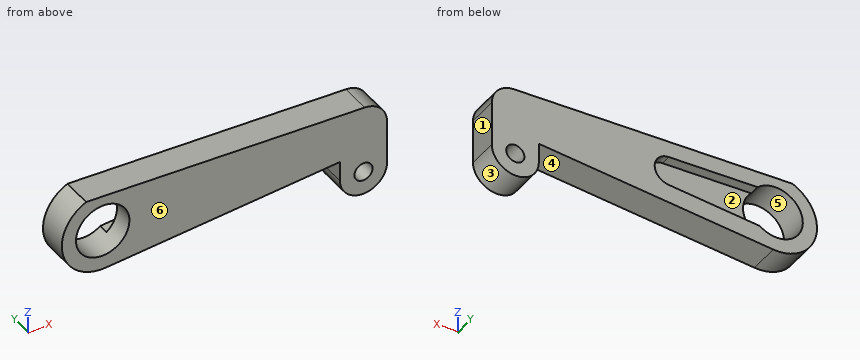
from build123d import *

# Parameters (mm, degrees)
BOSS_EXTRUDE1_START    = -1.35
BOSS_EXTRUDE1_DEPTH    = 1.35
SKETCH4_R              = 1.2192
BOSS_EXTRUDE2_DEPTH    = 4
BODY_DELETE1_OUTLINE_R = 2.45
BODY_DELETE1_DEPTH     = 4


# Read off the part's stored shape, not the designer's step: Body-Delete1
with BuildPart() as part:
    # Sketch2 → Revolve1 (revolve)
    with BuildSketch(Plane.XY, mode=Mode.PRIVATE) as revolve1_sk:
        Polygon((2.45, 0), (2.45, 2.25), (1.2, 2.25), (1.2, 3), (2.45, 3), (2.45, 4), (3.585, 4), (3.585, 0), align=None)
    revolve(revolve1_sk.sketch.rotate(Axis((0, 0, 0), (0, 1, 0)), 90), axis=Axis((0, 0, 0), (0, 1, 0)))

    # Sketch3 → Boss-Extrude1 (add)
    with BuildSketch(Plane(origin=(0, 4, 0), x_dir=(1, 0, 0), z_dir=(0, 1, 0)).offset(BOSS_EXTRUDE1_START)):
        with BuildLine():
            Line((2.174793094, 2.85), (14.4288372, 1.998853492))
            ThreePointArc((14.4288372, 1.998853492), (16.293577458, -0.019194273), (14.390517199, -2.001146508))
            Line((14.390517199, -2.001146508), (2.468243302, -2.6))
            ThreePointArc((2.468243302, -2.6), (3.579814485, 0.1927518), (2.174793094, 2.85))
        make_face()
    extrude(amount=BOSS_EXTRUDE1_DEPTH)


with BuildPart() as body_2:
    # Sketch4 → Boss-Extrude2 (new body)
    with BuildSketch(Plane(origin=(0, 0, 0), x_dir=(1, 0, 0), z_dir=(0, 1, 0))):
        with BuildLine():
            Line((0.380676568, 5.480639828), (31.845967375, 3.295110532))
            Line((31.845967375, 3.295110532), (31.845967375, 6))
            ThreePointArc((31.845967375, 6), (35, 9.154032625), (38.154032625, 6))
            Line((38.154032625, 6), (38.154032625, 0))
            ThreePointArc((38.154032625, 0), (37.285495002, -2.173576407), (35.158226963, -3.150061274))
            Line((35.158226963, -3.150061274), (-2.215454853, -5.027334022))
            ThreePointArc((-2.215454853, -5.027334022), (-5.333477425, 1.317704871), (0.380676568, 5.480639828))
        make_face()
        with Locations(Location((35, 6, 0), (0, 0, 270))):
            Circle(SKETCH4_R, mode=Mode.SUBTRACT)
    extrude(amount=BOSS_EXTRUDE2_DEPTH)

    # Combine1: cut part
    add(part.part, mode=Mode.SUBTRACT)

    # Body-Delete1 outline → Body-Delete1 (cut)
    with BuildSketch(Plane(origin=(0, 0, 0), x_dir=(1, 0, 0), z_dir=(0, 1, 0))):
        Circle(BODY_DELETE1_OUTLINE_R)
    extrude(amount=BODY_DELETE1_DEPTH, mode=Mode.SUBTRACT)


solid = body_2.part
Can you work these out from the model? Positions are in its coordinate system, mm. Face numbers are marked on the shaded views. A direction names the side the tool comes from. Give positions to 0.01 mm unless a question says otherwise; leave off trailing zeros. Order: outer loops, then holes, each group sorted by start corner. A loop starts at its lowest first (then second) coordinate and runs counter-clockwise, first axis right, second up. Notation, with made-up numbers: M -19,-17.75 L 18,-17.75 A17 cw 18,-1.75 Z; hole C 16.25,-27.5 d6. An arc over 180 degrees is marked long. Use a Markdown table: item, result. Add a question column.
Item 1: Suppose I cut it at C-C (x = 0). List the corners of the cut face in (y, z) for me (3 decimals), then the cut area to 3 significant figures.
Item 2: We'd pull the mould along X, two halves only. Please class the marked faces 3, 4, 5 and 6: +X half, -X half, draft (parallel to the pull), parting line (faces both ways), or undercut.
Item 3: If I drill on L1, parallel to X at y = 2.8, z = 0 (3 decimals); L2, parallel to X at y = 1.1, z = 0 (3 decimals); L3, parallel to Y at x = 7, z = 0.5, over which ranges is the centre line in solid material (lowest first)? Write a range as [from, to].
Item 4: Suppose I cut it at D-D (y = 1.2). List the corners of the cut face in (x, z) for me (3 decimals).
Item 5: For the marked faces 1 and 2, which set-ups out of +Z, -Z, +X, -X, +Y, -Y let a thin tool reach every point of the face, with its end or its side?
Item 6: Will these pins go through, and if not, where does the flat tip stop? pin 1 (1.5 mm diameter, centred on y = 1, z = -3, fed in from -X); pin 2 (1 mm diameter, centred on x = 12, y = 2, fed in from +Z); pin 3 (0.8 mm diameter, centred on y = 2.5, z = -4, fed in from -X).
Item 7: Suppose I cut it at B-B (z = 1.5). List the corners of the cut face in (x, y) for me.
Item 8: Suppose I cut it at A-A (y = 3.05). List the corners of the cut face in (x, z) for me (3 decimals).
Answer sheet:
| question | item | result |
|---|---|---|
| 1 | outline | M 0,-5.494 L 4,-5.494 L 4,-3.585 L 0,-3.585 Z; M 0,3.585 L 4,3.585 L 4,4.916 L 0,4.916 Z |
| 1 | area | 13.0 mm² |
| 2 | face 3 | parting line |
| 2 | face 4 | undercut |
| 2 | face 5 | undercut |
| 2 | face 6 | draft |
| 3 | L1 | x = [-5.494, -3.585], [16.294, 38.154] |
| 3 | L2 | x = [-5.494, -3.585], [3.585, 38.154] |
| 3 | L3 | y = [0, 2.65] |
| 4 | outline | M -2.215,5.027 A5.494 ccw 0.381,-5.481 L 31.846,-3.295 L 31.846,-6 A3.154 ccw 38.154,-6 L 38.154,0 A3.154 ccw 35.158,3.15 Z; hole C 0,0 d7.17; hole C 35,-6 d2.438 |
| 5 | face 1 | +Z, -Z, +X, +Y, -Y |
| 5 | face 2 | +Y |
| 6 | pin 1 | stops at x = -5.01 |
| 6 | pin 2 | stops at z = 4.34 |
| 6 | pin 3 | stops at x = -4.15 |
| 7 | outline | M -5.29,0 L -3.26,0 L -3.26,4 L -5.29,4 Z; M 3.26,0 L 37.77,0 L 37.77,4 L 15.62,4 L 15.62,2.65 L 3.26,2.65 Z |
| 8 | outline | M -2.215,5.027 A5.494 ccw 0.381,-5.481 L 31.846,-3.295 L 31.846,-6 A3.154 ccw 38.154,-6 L 38.154,0 A3.154 ccw 35.158,3.15 Z; hole M 2.175,-2.85 L 14.429,-1.999 A2.004 ccw 14.391,2.001 L 2.468,2.6 A3.585 ccw long Z; hole C 35,-6 d2.438 |
